Autodesk Inventor part; units mm, degrees
ref_plane "YZ Plane" through (0, 0, 0) normal (1, 0, 0) x (0, 1, 0)
ref_plane "XZ Plane" through (0, 0, 0) normal (0, 1, 0) x (-1, 0, 0)
ref_plane "XY Plane" through (0, 0, 0) normal (0, 0, 1) x (1, 0, 0)
sketch "Sketch1" plane through (0, 0, 0) normal (1, 0, 0) x (0, 1, 0)
  circle A0 centre (0, 0) radius 9
  dimension "d0" = 18
extrude "Extrusion1" add sketch "Sketch1" along normal blind 65
sketch "Sketch2" plane through (65, 0, 0) normal (1, 0, 0) x (0, 0, -1)
  circle A0 centre (0, 0) radius 6
  dimension "d3" = 12
extrude "Extrusion2" add sketch "Sketch2" along normal blind 0.2
fillet "Fillet1" radius 0.2 1 edges at (65.2, 0, 6)
fillet "Fillet2" radius 0.3 1 edges at (65, -9, 0)
fillet "Fillet3" radius 0.3 1 edges at (0, -9, 0)
sketch "Sketch3" plane through (0, 0, 0) normal (-1, 0, 0) x (0, 0, 1)
  circle A0 centre (0, 0) radius 5
  dimension "d9" = 10
extrude "Extrusion3" add sketch "Sketch3" along normal blind 0.7
fillet "Fillet4" radius 0.3 1 edges at (-0.7, 0, -5)
properties part number "18650-battery"
For this review, take the finished solid that the model builds, in its own axes (mm). A direction names the side the tool comes from. Give positions to 0.01 mm unless a question says otherwise; leave off trailing zeros. Loops run counter-clockwise (first coordinate to the right, second up) from the corner with the lowest first, then second, coordinate; pieces in that order, holes last. Notation, with made-up numbers: M -4.75,-21 L 11.25,-21 A19 ccw 11.25,-17 Z; hole C 8.5,10 d6. An arc over 180 degrees is marked long. Answer as a JSON object with one key per item and string values. Group by question number.
Q1. Add section A-A on x = 13.5. Give the boundary of the cut face in (y, z), and give its area (3 significant figures).
Q2. Tool access review of faces 3 (the flat face through (0, 4, -4)), 4 (the flat face through (-0.7, 0, 0)): name each direction out of +Z, -Z, +X, -X, +Y, -Y from which nothing blocks a thin tool from reaching the whole face with its end or side.
Q3. Insertion check: P1, Ø4, axis at x = 37, z = -5.5, coming from the -Y side; P2, Ø2, axis at x = 57, z = -0.5, coming from the -Y side; P3, Ø2, axis at x = 31, y = -2, coming from the -Z side; P4, Ø2, axis at x = 28.5, y = 4.5, coming from the +Z side. Each pin has a flat end and moves straight along its axis. Give the tip position at first contact, or say it passes through.
Q4. For probe 1 along X at (y, z) = (1.75, 5.5); probe 2 along X at (y, z) = (8.25, -1.5); probe 3 along Y at (x, z) = (46, 2), list the stretches that pass through material, from the lowest coordinate up. Write a range as [from, to].
Q5. Mouldability with a two-part tool opening along Z and no side actions: class faces 1 (the flat face through (65, 6, 2)), 2 (the cylindrical face through (-0.2, 4.88, -1.08)) as +Z half, -Z half, draft (parallel to the pull), parting line (faces both ways), or undercut.
Checked values:
{
 "1": {"outline": "C 0,0 d18", "area": "254 mm²"},
 "2": {"face 3": "-X", "face 4": "+Z, -Z, -X, +Y, -Y"},
 "3": {"P1": "y = -8.29", "P2": "y = -9", "P3": "z = -8.94", "P4": "z = 8.29"},
 "4": {"probe 1": "[0, 65.2]", "probe 2": "[0, 65]", "probe 3": "[-8.77, 8.77]"},
 "5": {"face 1": "draft", "face 2": "parting line"}
}
